Geometry check sheet. Reference: the model listing, model coordinates, mm. Face numbers are marked on the shaded views. Coordinates: 2 decimals unless noted, no trailing zeros. Order: outer loops, then holes, each group sorted by start corner. A loop starts at its lowest first (then second) coordinate and runs counter-clockwise, first axis right, second up. Notation, with made-up numbers: (54.5, 59) - (64.5, 59) arc R16 cw to (64.5, 81) - close; hole circle Ø11 at (-37, -27.5). An arc over 180 degrees is marked (long way). Return JSON: item names as keys, results as strings. Group by question number.
Item 1: Section check B-B on z = 13.5. Enter the section's corners in (x, y), then the cut area to 3 significant figures.
Item 2: Section check A-A on x = 0. Enter the section's corners in (y, z), then the cut area to 3 significant figures.
Item 3: Gauge pin test, flat end, axial feed: pin 1 (2 mm diameter, centred on x = 0.5, y = 0, fed in from +Z). Record the tip position at first contact, or that the pin passes through.
Item 4: Scan lines: probe 1 along Y at (x, z) = (0, 12.75); probe 2 along X at (y, z) = (0, 15.25); probe 3 along Y at (x, z) = (-1, 14.5). Record each from-to range of solid material in increasing order.
Item 5: Draft check along X on the marked faces 1, 2, 3 and 4. Enter one of: pulls with the +X half, pulls with the -X half, needs draft (parallel to the pull), parting line crosses it, or undercut.
Item 6: Section check C-C on y = -0.75. Enter the section's corners in (x, z), then the cut area to 3 significant figures.
Item 7: Section check D-D on z = 8.25. Enter the section's corners in (x, y).
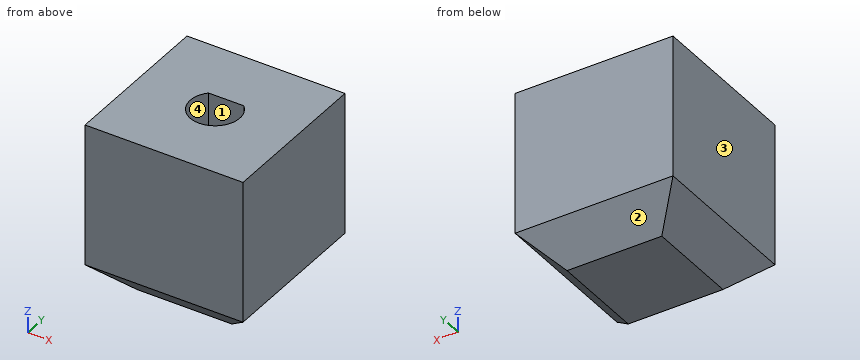
from build123d import *

# Parameters (mm, degrees)
BOX406008008_W     = 10
BOX406008008_H     = 10
BOX406008008_DEPTH = 19
CYLINDER079_R      = 1.57
CYLINDER079_DEPTH  = 17
BOX406008009_W     = 10
BOX406008009_H     = 10
BOX406008009_DEPTH = 11
CHAMFER004_SIZE    = 2


with BuildPart() as cube343:
    # Box406008008 → Box406008008 (new body)
    with BuildSketch(Plane(origin=(-5, 1.1, 1.5), x_dir=(1, 0, 0), z_dir=(0, 0, 1))):
        with Locations((5, 5)):
            Rectangle(BOX406008008_W, BOX406008008_H)
    extrude(amount=BOX406008008_DEPTH)


with BuildPart() as motor_shaft_hole:
    # Cylinder079 → Cylinder079 (new body)
    with BuildSketch(Plane.XY.offset(9)):
        Circle(CYLINDER079_R)
    extrude(amount=CYLINDER079_DEPTH)

    # Cut064: cut Cube343
    add(cube343.part, mode=Mode.SUBTRACT)


with BuildPart() as square_peg001:
    # Box406008009 → Box406008009 (new body)
    with BuildSketch(Plane(origin=(-5, -5, 7), x_dir=(1, 0, 0), z_dir=(0, 0, 1))):
        with Locations((5, 5)):
            Rectangle(BOX406008009_W, BOX406008009_H)
    extrude(amount=BOX406008009_DEPTH)

    # Cut065: cut Motor Shaft Hole
    add(motor_shaft_hole.part, mode=Mode.SUBTRACT)

    # Chamfer004
    chamfer004_edges = [square_peg001.edges().sort_by_distance(p)[0] for p in [
        (-5, 0, 7),
        (0, -5, 7),
        (0, 5, 7),
        (5, 0, 7),
    ]]
    chamfer(chamfer004_edges, length=CHAMFER004_SIZE)


solid = square_peg001.part
Computed:
{
 "1": {"outline": "(-5, -5) - (5, -5) - (5, 5) - (-5, 5) - close; hole (-1.12, 1.1) arc R1.57 ccw (long way) to (1.12, 1.1) - close", "area": "93.0 mm²"},
 "2": {"outline": "(-5, 9) - (-3, 7) - (3, 7) - (5, 9) - (5, 18) - (1.1, 18) - (1.1, 9) - (-1.57, 9) - (-1.57, 18) - (-5, 18) - close", "area": "82.0 mm²"},
 "3": {"pin 1": "stops at z = 9"},
 "4": {"probe 1": "y = -5 to -1.57, 1.1 to 5", "probe 2": "x = -5 to -1.57, 1.57 to 5", "probe 3": "y = -5 to -1.21, 1.1 to 5"},
 "5": {"face 1": "undercut", "face 2": "needs draft", "face 3": "pulls with the -X half", "face 4": "undercut"},
 "6": {"outline": "(-5, 9) - (-3, 7) - (3, 7) - (5, 9) - (5, 18) - (1.38, 18) - (1.38, 9) - (-1.38, 9) - (-1.38, 18) - (-5, 18) - close", "area": "81.2 mm²"},
 "7": {"outline": "(-4.25, -4.25) - (4.25, -4.25) - (4.25, 4.25) - (-4.25, 4.25) - close"}
}
